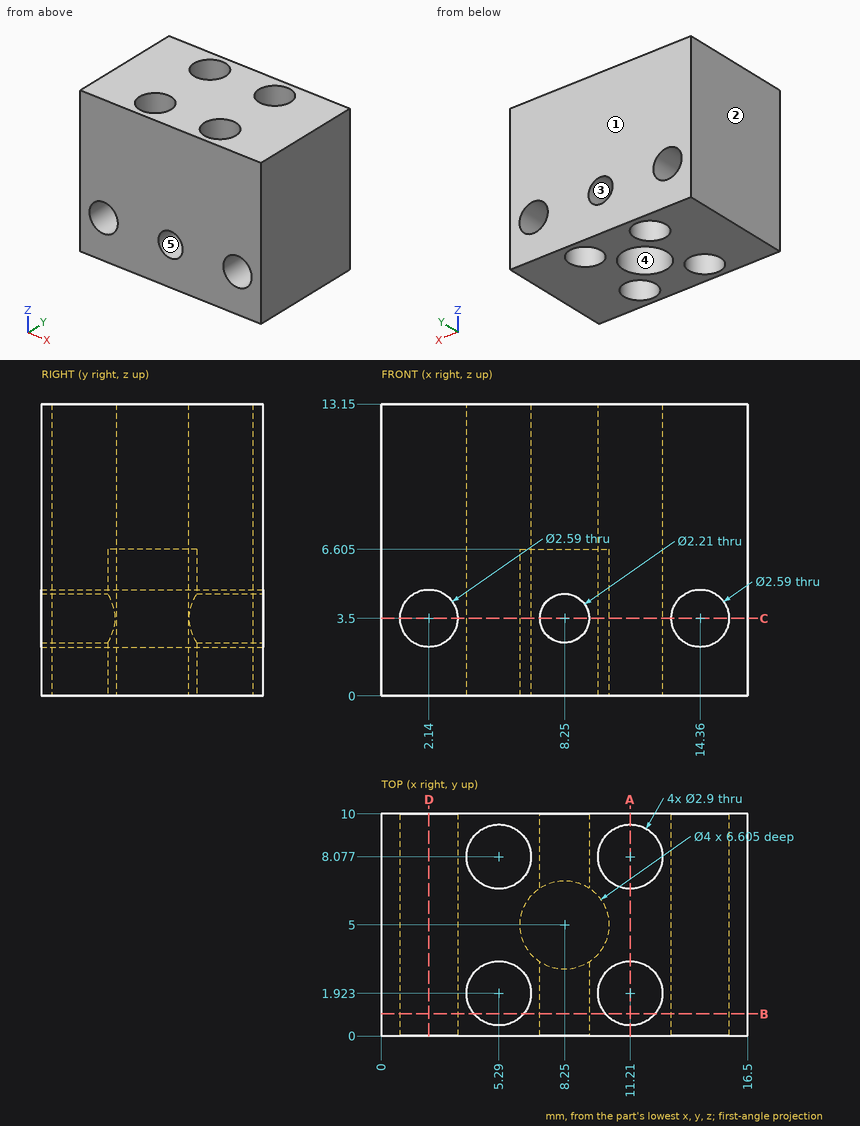
Study the drawing (mm; zero at the part's minimum x, y, z) and answer. A direction names the side the tool comes from. Round coordinates to 2 decimals unless told otherwise and drop trailing zeros. Order: outer loops, then holes, each group sorted by start corner. A loop starts at its lowest first (then second) coordinate and runs counter-clockwise, first axis right, second up. Notation, with made-up numbers: (-9, 86.25) - (-2, 86.25) arc R17 cw to (-2, 111.25) - close; hole circle Ø3 at (12, -8.5). An arc over 180 degrees is marked (long way). Use one line per item in the form item = value. Start each with the question number.
(1) The part is cut by section A-A (x = 11.21). Give the vertices of the cut face in (y, z), then the cut area to 3 significant figures.
(2) Determine the mould class of the marked faces 1, 2 and 3 for opening direction X: +X half, -X half, draft (parallel to the pull), parting line (faces both ways), or undercut.
(3) A flat-ended cylindrical pin translates along its axis: pin 1 Ø2.5 at (x, z) = (14.36, 3.5) entering from +Y. Find the tip coordinate at first contact, or state that the pin passes through.
(4) The part is cut by section B-B (y = 1). Count the separate pieces of the cut face and the enclosed holes in it, then the cut area to 3 significant figures.
(5) Find the intervals of material crossed by line 1 along X through (y, z) = (2, 1); line 2 along Y through (x, z) = (5.29, 4.5); line 3 along Z through (x, y) = (8.25, 1.5) (3 decimals), in increasing order. Write a range as from..to.
(6) The part is cut by section D-D (x = 2.14). Give the vertices of the cut face in (y, z) (3 decimals).
(7) The part is cut by section C-C (z = 3.5). Give the vertices of the cut face in (x, y) (3 decimals), then the cut area to 3 significant figures.
(8) For the marked faces 4 and 5, determine the directions among +Z, -Z, +X, -X, +Y, -Y from which every point of the face is accessible in a straight line to the end or side of a thin tool.
Checked values:
q1.outline = (0, 0) - (0.47, 0) - (0.47, 13.15) - (0, 13.15) - close; (3.37, 0) - (6.63, 0) - (6.63, 13.15) - (3.37, 13.15) - close; (9.53, 0) - (10, 0) - (10, 13.15) - (9.53, 13.15) - close
q1.area = 55.2 mm^2
q2.face_1 = draft
q2.face_2 = -X half
q2.face_3 = undercut
q3.pin_1 = through
q4.separate_pieces = 3
q4.enclosed_holes = 3
q4.area = 144 mm^2
q5.line_1 = 0..3.84, 6.74..9.76, 12.66..16.5
q5.line_2 = 0..0.47, 3.37..6.63, 9.53..10
q5.line_3 = 0..2.395, 4.605..13.15
q6.outline = (0, 0) - (10, 0) - (10, 2.205) - (0, 2.205) - close; (0, 4.795) - (10, 4.795) - (10, 13.15) - (0, 13.15) - close
q7.outline = (0, 0) - (0.845, 0) - (0.845, 10) - (0, 10) - close; (3.435, 0) - (7.145, 0) - (7.145, 3.333) arc R2 cw to (7.145, 6.667) - (7.145, 10) - (3.435, 10) - close; (9.355, 0) - (13.065, 0) - (13.065, 10) - (9.355, 10) - (9.355, 6.667) arc R2 cw to (9.355, 3.333) - close; (15.655, 0) - (16.5, 0) - (16.5, 10) - (15.655, 10) - close; hole circle Ø2.9 at (5.29, 1.923); hole circle Ø2.9 at (5.29, 8.077); hole circle Ø2.9 at (11.21, 1.923); hole circle Ø2.9 at (11.21, 8.077)
q7.area = 60.5 mm^2
q8.face_4 = -Z
q8.face_5 = +Y, -Y
